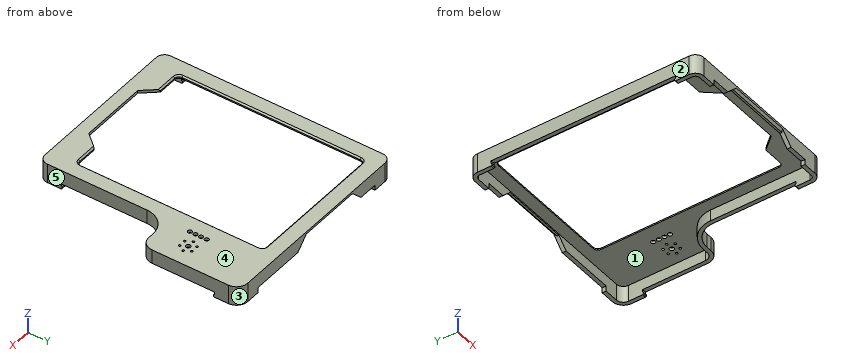
```python
from build123d import *

# Parameters (mm, degrees)
PAD007_DEPTH    = 10
POCKET006_DEPTH = 8
POCKET007_DEPTH = 2
SKETCH022_R     = 1.5
SKETCH022_R_2   = 1.6
SKETCH022_R_3   = 0.8
POCKET009_DEPTH = 2
POCKET010_DEPTH = 162.801
PAD011_DEPTH    = 3.8
SKETCH045_W     = 2.8
SKETCH045_H     = 2
SKETCH046_W     = 2.8
SKETCH046_H     = 1.2
SKETCH047_W     = 2.8
SKETCH047_H     = 2
SKETCH048_W     = 2.8
SKETCH048_H     = 1.2
SKETCH049_W     = 2.8
SKETCH049_H     = 2
SKETCH050_W     = 2.8
SKETCH050_H     = 1.2
SKETCH051_W     = 2.8
SKETCH051_H     = 2
SKETCH052_W     = 2.8
SKETCH052_H     = 1.2
CHAMFER003_SIZE = 1.4
CHAMFER004_SIZE = 1


with BuildPart() as part:
    # Sketch014 → Pad007 (new body)
    with BuildSketch(Plane.XY):
        with BuildLine():
            Line((-54.5, 81.4), (80, 81.4))
            ThreePointArc((88, 73.4), (85.656854, 79.056854), (80, 81.4))
            Line((88, 73.4), (88, 19))
            ThreePointArc((80, 11), (85.656854, 13.343146), (88, 19))
            Line((76, 11), (80, 11))
            ThreePointArc((76, 11), (65.039845, 6.460155), (60.5, -4.5))
            Line((60.5, -75.4), (60.5, -4.5))
            ThreePointArc((54.5, -81.4), (58.742641, -79.642641), (60.5, -75.4))
            Line((54.5, -81.4), (-54.5, -81.4))
            ThreePointArc((-60.5, -75.4), (-58.742641, -79.642641), (-54.5, -81.4))
            Line((-60.5, -75.4), (-60.5, 75.4))
            ThreePointArc((-54.5, 81.4), (-58.742641, 79.642641), (-60.5, 75.4))
        make_face()
    extrude(amount=-PAD007_DEPTH)

    # Sketch017 (on Face14 of Pad007) → Pocket006 (cut)
    with BuildSketch(Plane(origin=(0, 0, -10), x_dir=(1, 0, 0), z_dir=(0, 0, -1))):
        with BuildLine():
            Line((-54.7, 78.6), (54.7, 78.6))
            ThreePointArc((57.7, 75.6), (56.82132, 77.72132), (54.7, 78.6))
            Line((57.7, 4.7), (57.7, 75.6))
            ThreePointArc((57.7, 4.7), (63.118525, -8.381475), (76.2, -13.8))
            Line((80.2, -13.8), (76.2, -13.8))
            ThreePointArc((85.2, -18.8), (83.735534, -15.264466), (80.2, -13.8))
            Line((85.2, -18.8), (85.2, -73.6))
            ThreePointArc((80.2, -78.6), (83.735534, -77.135534), (85.2, -73.6))
            Line((80.2, -78.6), (-54.7, -78.6))
            ThreePointArc((-57.7, -75.6), (-56.82132, -77.72132), (-54.7, -78.6))
            Line((-57.7, -75.6), (-57.7, 75.6))
            ThreePointArc((-54.7, 78.6), (-56.82132, 77.72132), (-57.7, 75.6))
        make_face()
    extrude(amount=-POCKET006_DEPTH, mode=Mode.SUBTRACT)

    # Sketch018 (on Face4 of Pocket006) → Pocket007 (cut)
    with BuildSketch(Plane.XY):
        with BuildLine():
            Line((-46.5, 70.4), (46.5, 70.4))
            ThreePointArc((49.5, 67.4), (48.62132, 69.52132), (46.5, 70.4))
            Line((49.5, 67.4), (49.5, -59.4))
            ThreePointArc((46.5, -62.4), (48.62132, -61.52132), (49.5, -59.4))
            Line((46.5, -62.4), (32.5, -62.4))
            Line((32.5, -62.4), (24, -72.4))
            Line((24, -72.4), (-24, -72.4))
            Line((-24, -72.4), (-32.5, -62.4))
            Line((-32.5, -62.4), (-46.5, -62.4))
            ThreePointArc((-49.5, -59.4), (-48.62132, -61.52132), (-46.5, -62.4))
            Line((-49.5, -59.4), (-49.5, 67.4))
            ThreePointArc((-46.5, 70.4), (-48.62132, 69.52132), (-49.5, 67.4))
        make_face()
    extrude(amount=-POCKET007_DEPTH, mode=Mode.SUBTRACT)

    # Sketch022 (on Face4 of Pocket007) → Pocket009 (cut)
    with BuildSketch(Plane.XY):
        with Locations((61.8, 39)):
            Circle(SKETCH022_R)
        with Locations((61.8, 35)):
            Circle(SKETCH022_R)
        with Locations((61.8, 31)):
            Circle(SKETCH022_R)
        with Locations((61.8, 27)):
            Circle(SKETCH022_R)
        with Locations((73, 34)):
            Circle(SKETCH022_R_2)
        with Locations((70.5, 38.330127)):
            Circle(SKETCH022_R_3)
        with Locations((75.5, 38.330127)):
            Circle(SKETCH022_R_3)
        with Locations((78, 34)):
            Circle(SKETCH022_R_3)
        with Locations((75.5, 29.669873)):
            Circle(SKETCH022_R_3)
        with Locations((70.5, 29.669873)):
            Circle(SKETCH022_R_3)
        with Locations((68, 34)):
            Circle(SKETCH022_R_3)
    extrude(amount=-POCKET009_DEPTH, mode=Mode.SUBTRACT)

    # Sketch023 (on Face7 of Pocket009) → Pocket010 (cut, through all)
    with BuildSketch(Plane(origin=(0, 81.4, 0), x_dir=(-1, 0, 0), z_dir=(0, 1, 0))):
        Polygon((-24, -3), (24, -3), (31, -10), (-31, -10), align=None)
    extrude(amount=-POCKET010_DEPTH, mode=Mode.SUBTRACT)

    # Sketch026 (on Face5 of Pocket010) → Pad011 (join)
    with BuildSketch(Plane(origin=(0, 0, -10), x_dir=(1, 0, 0), z_dir=(0, 0, -1))):
        with BuildLine():
            Line((-54.5, 81.4), (-44.7, 81.4))
            Line((-44.7, 81.4), (-44.7, 78.6))
            Line((-54.7, 78.6), (-44.7, 78.6))
            ThreePointArc((-54.7, 78.6), (-56.82132, 77.72132), (-57.7, 75.6))
            Line((-57.7, 65.6), (-57.7, 75.6))
            Line((-57.7, 65.6), (-60.5, 65.6))
            Line((-60.5, 65.6), (-60.5, 75.4))
            ThreePointArc((-54.5, 81.4), (-58.742641, 79.642641), (-60.5, 75.4))
        make_face()
        with BuildLine():
            Line((54.5, 81.4), (44.7, 81.4))
            Line((44.7, 81.4), (44.7, 78.6))
            Line((54.7, 78.6), (44.7, 78.6))
            ThreePointArc((57.7, 75.6), (56.82132, 77.72132), (54.7, 78.6))
            Line((57.7, 65.6), (57.7, 75.6))
            Line((57.7, 65.6), (60.5, 65.6))
            Line((60.5, 65.6), (60.5, 75.4))
            ThreePointArc((60.5, 75.4), (58.742641, 79.642641), (54.5, 81.4))
        make_face()
        with BuildLine():
            Line((-54.5, -81.4), (-44.7, -81.4))
            Line((-44.7, -81.4), (-44.7, -78.6))
            Line((-54.7, -78.6), (-44.7, -78.6))
            ThreePointArc((-57.7, -75.6), (-56.82132, -77.72132), (-54.7, -78.6))
            Line((-57.7, -65.6), (-57.7, -75.6))
            Line((-57.7, -65.6), (-60.5, -65.6))
            Line((-60.5, -65.6), (-60.5, -75.4))
            ThreePointArc((-60.5, -75.4), (-58.742641, -79.642641), (-54.5, -81.4))
        make_face()
        with BuildLine():
            Line((80, -81.4), (70.2, -81.4))
            Line((70.2, -81.4), (70.2, -78.6))
            Line((80.2, -78.6), (70.2, -78.6))
            ThreePointArc((80.2, -78.6), (83.735534, -77.135534), (85.2, -73.6))
            Line((85.2, -63.6), (85.2, -73.6))
            Line((85.2, -63.6), (88, -63.6))
            Line((88, -63.6), (88, -73.4))
            ThreePointArc((80, -81.4), (85.656854, -79.056854), (88, -73.4))
        make_face()
    extrude(amount=PAD011_DEPTH)

    # Sketch045 (on DatumPlane) → AdditiveLoft section 0
    with BuildSketch(Plane(origin=(0, -65.6, 0), x_dir=(-1, 0, 0), z_dir=(0, 1, 0))):
        with Locations((-59.1, -12.8)):
            Rectangle(SKETCH045_W, SKETCH045_H)
    # Sketch046 (on DatumPlane) → AdditiveLoft section 1
    with BuildSketch(Plane(origin=(0, -65, 0), x_dir=(-1, 0, 0), z_dir=(0, 1, 0))):
        with Locations((-59.1, -12.8)):
            Rectangle(SKETCH046_W, SKETCH046_H)
    loft()

    # Sketch047 (on DatumPlane) → AdditiveLoft001 section 0
    with BuildSketch(Plane(origin=(0, -65.6, 0), x_dir=(-1, 0, 0), z_dir=(0, 1, 0))):
        with Locations((59.1, -12.8)):
            Rectangle(SKETCH047_W, SKETCH047_H)
    # Sketch048 (on DatumPlane) → AdditiveLoft001 section 1
    with BuildSketch(Plane(origin=(0, -65, 0), x_dir=(-1, 0, 0), z_dir=(0, 1, 0))):
        with Locations((59.1, -12.8)):
            Rectangle(SKETCH048_W, SKETCH048_H)
    loft()

    # Sketch049 (on DatumPlane) → AdditiveLoft002 section 0
    with BuildSketch(Plane.XZ.offset(-65.6)):
        with Locations((-59.1, -12.8)):
            Rectangle(SKETCH049_W, SKETCH049_H)
    # Sketch050 (on DatumPlane) → AdditiveLoft002 section 1
    with BuildSketch(Plane.XZ.offset(-65)):
        with Locations((-59.1, -12.8)):
            Rectangle(SKETCH050_W, SKETCH050_H)
    loft()

    # Sketch051 (on DatumPlane) → AdditiveLoft003 section 0
    with BuildSketch(Plane.XZ.offset(-63.6)):
        with Locations((86.6, -12.8)):
            Rectangle(SKETCH051_W, SKETCH051_H)
    # Sketch052 (on DatumPlane) → AdditiveLoft003 section 1
    with BuildSketch(Plane.XZ.offset(-63)):
        with Locations((86.6, -12.8)):
            Rectangle(SKETCH052_W, SKETCH052_H)
    loft()

    # Chamfer003
    chamfer003_edges = [part.edges().sort_by_distance(p)[0] for p in [
        (0, -81.4, -3),
        (0, 81.4, -3),
    ]]
    chamfer(chamfer003_edges, length=CHAMFER003_SIZE)

    # Chamfer004
    chamfer004_edges = [part.edges().sort_by_distance(p)[0] for p in [
        (-49.5, 4, 0),
    ]]
    chamfer(chamfer004_edges, length=CHAMFER004_SIZE)


with BuildPart() as part_1:
    # Body002 placement: moved
    add(part.part.moved(Location((0, 0, 21))))


solid = part_1.part
```
Design review of the part built by this model. Coordinates are the model's own, in mm. Face numbers are marked on the shaded views. A direction names the side the tool comes from. Round coordinates to 2 decimals unless told otherwise and drop trailing zeros. Order: outer loops, then holes, each group sorted by start corner. A loop starts at its lowest first (then second) coordinate and runs counter-clockwise, first axis right, second up. Notation, with made-up numbers: M -5.5,31 L 24.5,31 A13 ccw 24.5,47 Z; hole C 5,3 d11. An arc over 180 degrees is marked long. Put each result on its own line as item: value.
Q1. Insertion check: pin 1 Ø0.6 at (x, z) = (58.5, 8.5) entering from +Y; pin 2 Ø0.7 at (x, y) = (6, -79.5) entering from -Z; pin 3 Ø2 at (y, z) = (80.5, 8.5) entering from -X; pin 4 Ø5 at (x, y) = (48.5, 7) entering from +Z. Each pin has a flat end and moves straight along its axis. Give the tip position at first contact, or say it passes through.
Reported:
pin 1: y = -65
pin 2: z = 18
pin 3: x = -58.88
pin 4: z = 21
Q2. Draft analysis for pull direction Y (two halves, no side actions). For the marked faces 1, 2 and 3, state which applies: released by +Y, released by -Y, zero draft, split by the parting line, or undercut.
Reported:
face 1: undercut
face 2: zero draft
face 3: released by +Y
Q3. Consider section A-A (x = -19.5). State the section outline as (y, z) points.
Reported:
outline: M -81.4,19.4 L -80,18 L -78.6,18 L -78.6,19 L -72.4,19 L -72.4,21 L -81.4,21 Z; M 70.4,19 L 78.6,19 L 78.6,18 L 80,18 L 81.4,19.4 L 81.4,21 L 71.4,21 L 70.4,20 Z
Q4. Consider section D-D (y = 46). State the section outline as (x, z) points.
Reported:
outline: M -60.5,11 L -57.7,11 L -57.7,19 L -49.5,19 L -49.5,20 L -50.5,21 L -60.5,21 Z; M 49.5,19 L 85.2,19 L 85.2,11 L 88,11 L 88,21 L 50.5,21 L 49.5,20 Z
Q5. Consider section B-B (y = -43.5). State the section outline as (x, z) points, and give its area (3 significant figures).
Reported:
outline: M -60.5,11 L -57.7,11 L -57.7,19 L -49.5,19 L -49.5,20 L -50.5,21 L -60.5,21 Z; M 49.5,19 L 57.7,19 L 57.7,11 L 60.5,11 L 60.5,21 L 50.5,21 L 49.5,20 Z
area: 87.8 mm²
Q6. Machinability: for the marked faces 4 and 5, which of the approach directions +Z, -Z, +X, -X, +Y, -Y give a long, thin tool a straight path to every point of the face, cutting with its end or side? Answer none if there is none.
Reported:
face 4: +Z, +X, -X, +Y, -Y
face 5: +Z, -Z, +X, -Y
Q7. To check wall thickness, follow line 1 (X direction, y = -15, z = 15); line 2 (Y direction, x = 61.8, z = 20.55); line 3 (X direction, y = 24.5, z = 19.5). State the ranges of each line that lie inside material, in increasing order.
Reported:
line 1: -60.5 to -57.7, 57.7 to 60.5
line 2: 1.71 to 25.5, 28.5 to 29.5, 32.5 to 33.5, 36.5 to 37.5, 40.5 to 81.4
line 3: -60.5 to -49.5, 49.5 to 88
